Autodesk Inventor part; units mm, degrees
ref_plane "YZ Plane" through (0, 0, 0) normal (1, 0, 0) x (0, 1, 0)
ref_plane "XZ Plane" through (0, 0, 0) normal (0, 1, 0) x (-1, 0, 0)
ref_plane "XY Plane" through (0, 0, 0) normal (0, 0, 1) x (1, 0, 0)
sketch "Sketch1" plane through (0, 0, 0) normal (0, 0, 1) x (1, 0, 0)
  circle A0 centre (0, 0) radius 4
  circle A1 centre (0, 0) radius 6
  dimension "d0" = 8
  dimension "d1" = 12
extrude "Extrusion1" add sketch "Sketch1" along normal blind 6
sketch "Sketch2" plane through (0, 0, 6) normal (0, 0, 1) x (1, 0, 0)
  line L0 (-4.5, -4.5) -> (4.5, -4.5)
  line L1 (4.5, -4.5) -> (4.5, 4.5)
  line L2 (4.5, 4.5) -> (-4.5, 4.5)
  line L3 (-4.5, 4.5) -> (-4.5, -4.5)
  line L4 (-4.5, -4.5) -> (4.5, 4.5) construction
  line L5 (4.5, -4.5) -> (-4.5, 4.5) construction
  point P0 (0, 0)
  dimension "d4" = 9
  dimension "d5" = 9
extrude "Extrusion2" add sketch "Sketch2" along normal blind 3
fillet "Fillet1" radius 2 4 edges at (-4.5, -4.5, 7.5) (-4.5, 4.5, 7.5) (4.5, 4.5, 7.5) (4.5, -4.5, 7.5)
thread "Thread1"
properties part number "Nakrętka na belkę" material "Aluminum 6061"
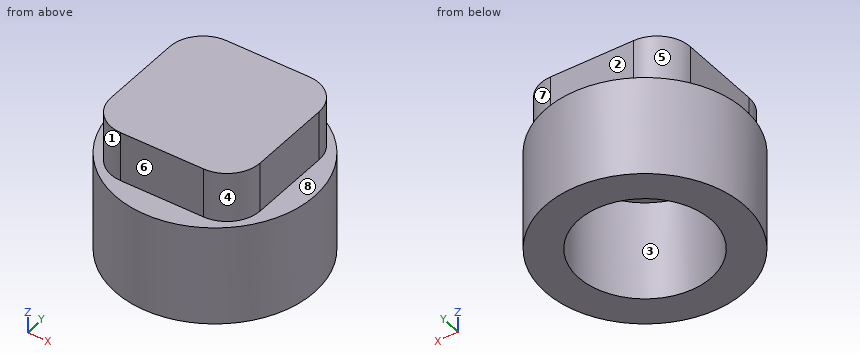
Work out the finished part from the listing and answer in its coordinate system (mm). Face numbers are marked on the shaded views. A direction names the side the tool comes from. Give positions to 0.01 mm unless a question says otherwise; leave off trailing zeros. Order: outer loops, then holes, each group sorted by start corner. A loop starts at its lowest first (then second) coordinate and runs counter-clockwise, first axis right, second up. Notation, with made-up numbers: M 1,74.5 L 30,74.5 A14 cw 30,81.5 Z; hole C 89.5,75 d8. An arc over 180 degrees is marked long. Return JSON: item names as keys, results as strings.
Q1. Find section D-D, the plane z = 3. Write down the section's boundary in (x, y), and give its area (3 significant figures).
Answer below:
{"outline": "C 0,0 d12; hole C 0,0 d8", "area": "62.8 mm^2"}
Q2. The mould has two halves that part along X. Classify the marked faces 1, 2, 3 and 4: pulls with the +X half, pulls with the -X half, needs draft (parallel to the pull), parting line crosses it, or undercut.
Answer below:
{"face 1": "pulls with the -X half", "face 2": "needs draft", "face 3": "undercut", "face 4": "pulls with the +X half"}
Q3. Each of these flat-tipped pins is pushed along its axis until it touches: pin 1 (0.9 mm diameter, centred on x = 1, z = 7.5, fed in from -Y); pin 2 (1.5 mm diameter, centred on y = -0.5, z = 7.5, fed in from +X); pin 3 (4 mm diameter, centred on x = -4, z = 5.5, fed in from +Y). Where does it stop, or does it pass through?
Answer below:
{"pin 1": "stops at y = -4.5", "pin 2": "stops at x = 4.5", "pin 3": "stops at y = 5.66"}
Q4. Find section A-A, the plane x = 0. Write down the section's boundary in (y, z).
Answer below:
{"outline": "M -6,0 L -4,0 L -4,6 L 4,6 L 4,0 L 6,0 L 6,6 L 4.5,6 L 4.5,9 L -4.5,9 L -4.5,6 L -6,6 Z"}
Q5. Find section C-C, the plane z = 7.75. Write down the section's boundary in (x, y), and give its area (3 significant figures).
Answer below:
{"outline": "M -4.5,-2.5 A2 ccw -2.5,-4.5 L 2.5,-4.5 A2 ccw 4.5,-2.5 L 4.5,2.5 A2 ccw 2.5,4.5 L -2.5,4.5 A2 ccw -4.5,2.5 Z", "area": "77.6 mm^2"}
Q6. Which of the six approach directions +Z, -Z, +X, -X, +Y, -Y give full straight-line access (tool end or side, diameter ignored) to the marked faces 5, 6, 7 and 8?
Answer below:
{"face 5": "+Z, -X, +Y", "face 6": "+Z, +X, -X, -Y", "face 7": "+Z, +X, +Y", "face 8": "+Z"}
Q7. Find the intervals of material crossed by line 1 along Y through (x, z) = (0, 4.1); line 2 along Z through (x, y) = (1.25, 0.25); line 3 along Z through (x, y) = (-4.5, -3.25), in increasing order. Write a range as [from, to].
Answer below:
{"line 1": "y = [-6, -4], [4, 6]", "line 2": "z = [6, 9]", "line 3": "z = [0, 6]"}
